Verification items for the finished model (mm, model axes). Face numbers are marked on the shaded views. A direction names the side the tool comes from. Give positions to 0.01 mm unless a question says otherwise; leave off trailing zeros. Order: outer loops, then holes, each group sorted by start corner. A loop starts at its lowest first (then second) coordinate and runs counter-clockwise, first axis right, second up. Notation, with made-up numbers: (66, 86.25) -> (82, 86.25) arc R27 cw to (82, 120.25) -> close; hole circle Ø8 at (67.25, 5.5). An arc over 180 degrees is marked (long way). Return JSON: item names as keys, results as strings. Group by question number.
(1) Cross-section at D-D on y = -50. Enter the section's corners in (x, z).
(2) Release check for a two-part mould opening along X. For the marked faces 1, 2 and 3 record: pulls with the +X half, pulls with the -X half, needs draft (parallel to the pull), parting line crosses it, or undercut.
(3) Cross-section at B-B on x = 0. Enter the section's corners in (y, z), then the cut area to 3 significant figures.
(4) Cross-section at C-C on z = -43. Enter the section's corners in (x, y), then the cut area to 3 significant figures.
(5) Thickness scan on line 1 along Y through (x, z) = (0, 1.5); line 2 along Z through (x, y) = (-19, 23.5); line 3 along Z through (x, y) = (17, 21). Record the ranges inside material, lowest first.
(6) Depth check by flat-ended pin: pin 1 Ø1.2 at (x, z) = (0, -43) entering from +Y; pin 2 Ø12 at (x, z) = (-18.5, -20.5) entering from -Y; pin 3 Ø8 at (x, z) = (15, -29.5) entering from +Y; pin 4 Ø11 at (x, y) = (7.5, 2.5) entering from +Z. Enter the tip coordinate at first touch or a pass-through.
(7) Cross-section at A-A on z = -1.5. Enter the section's corners in (x, y), then the cut area to 3 significant figures.
(8) Tool access check on the marked faces 4, 5, 6, 7 and 8. Record the directions out of +Z, -Z, +X, -X, +Y, -Y that give a thin tool (end or side, any length) a straight path to the whole face; none if there is none.
from build123d import *

# Parameters (mm, degrees)
F0_R      = 3.25
F1_DEPTH  = 50
F2_W      = 120.846782
F2_H      = 139.899194
F2_R      = 27.5
F3_DEPTH  = 45
F5_DEPTH  = 20
F7_DEPTH  = 10
F8_R      = 3.25
F8_R_2    = 27.5
F9_DEPTH  = 45
F10_W     = 122.298393
F10_H     = 98.165326
F10_R     = 5
F11_DEPTH = 20
F12_W     = 4
F12_H     = 52
F13_DEPTH = 20


with BuildPart() as f1:
    # F0 (on Top) → F1 (new body, symmetric)
    with BuildSketch(Plane.XY):
        with BuildLine():
            ThreePointArc((26.318053, -14.400002), (29.064941, -7.431635), (30, 0))
            ThreePointArc((30, 0), (29.064941, 7.431635), (26.318053, 14.400002))
            ThreePointArc((26.318053, 14.400002), (0, 30), (-26.318053, 14.400002))
            ThreePointArc((-26.318053, 14.400002), (-30, 0), (-26.318053, -14.400002))
            ThreePointArc((-26.318053, -14.400002), (0, -30), (26.318053, -14.400002))
        make_face()
        with BuildLine():
            ThreePointArc((-26.318053, 14.400002), (0, 30), (26.318053, 14.400002))
            Line((26.318053, 14.400002), (5.263611, 52.88))
            ThreePointArc((5.263611, 52.88), (5.812988, 51.486327), (6, 50))
            ThreePointArc((6, 50), (-1.486327, 44.187012), (-5.263611, 52.88))
            Line((-5.263611, 52.88), (-26.318053, 14.400002))
        make_face()
        with BuildLine():
            Line((5.263611, -52.88), (26.318053, -14.400002))
            ThreePointArc((26.318053, -14.400002), (0, -30), (-26.318053, -14.400002))
            Line((-26.318053, -14.400002), (-5.263611, -52.88))
            ThreePointArc((-5.263611, -52.88), (-1.486327, -44.187012), (6, -50))
            ThreePointArc((6, -50), (5.812988, -51.486327), (5.263611, -52.88))
        make_face()
        with BuildLine():
            ThreePointArc((6, 50), (5.812988, 51.486327), (5.263611, 52.88))
            ThreePointArc((5.263611, 52.88), (0, 56), (-5.263611, 52.88))
            ThreePointArc((-5.263611, 52.88), (-1.486327, 44.187012), (6, 50))
        make_face()
        with Locations((0, 50)):
            Circle(F0_R, mode=Mode.SUBTRACT)
        with BuildLine():
            ThreePointArc((-5.263611, -52.88), (0, -56), (5.263611, -52.88))
            ThreePointArc((5.263611, -52.88), (5.812988, -51.486327), (6, -50))
            ThreePointArc((6, -50), (-1.486327, -44.187012), (-5.263611, -52.88))
        make_face()
        with Locations((0, -50)):
            Circle(F0_R, mode=Mode.SUBTRACT)
    extrude(amount=F1_DEPTH, both=True)

    # F2 (on face) → F3 (cut)
    with BuildSketch(Plane.XY.offset(50)):
        with Locations((4.808469, 0)):
            Rectangle(F2_W, F2_H)
        Circle(F2_R, mode=Mode.SUBTRACT)
    extrude(amount=-F3_DEPTH, mode=Mode.SUBTRACT)

    # F4 (on face) → F5 (cut)
    with BuildSketch(Plane.XY.offset(50)):
        with BuildLine():
            Line((-2.5, 16.312995), (-2.5, 38.387493))
            ThreePointArc((-2.5, 38.387493), (-38.468814, 0), (-2.5, -38.387493))
            Line((-2.5, -38.387493), (-2.5, -16.312995))
            ThreePointArc((-2.5, -16.312995), (-16.503448, 0), (-2.5, 16.312995))
        make_face()
        with BuildLine():
            ThreePointArc((2.5, -38.387493), (38.468814, 0), (2.5, 38.387493))
            Line((2.5, 38.387493), (2.5, 16.312995))
            ThreePointArc((2.5, 16.312995), (16.503448, 0), (2.5, -16.312995))
            Line((2.5, -16.312995), (2.5, -38.387493))
        make_face()
    extrude(amount=-F5_DEPTH, mode=Mode.SUBTRACT)

    # F6 (on face) → F7 (cut)
    with BuildSketch(Plane.XY.offset(50)):
        with BuildLine():
            ThreePointArc((2.5, 5.454356), (5.049752, 3.24037), (6, 0))
            ThreePointArc((6, 0), (5.049752, -3.24037), (2.5, -5.454356))
            Line((2.5, -5.454356), (2.5, -22.150979))
            ThreePointArc((2.5, -22.150979), (22.29161, 0), (2.5, 22.150979))
            Line((2.5, 22.150979), (2.5, 5.454356))
        make_face()
        with BuildLine():
            ThreePointArc((-2.5, -5.454356), (-6, 0), (-2.5, 5.454356))
            Line((-2.5, 5.454356), (-2.5, 22.150979))
            ThreePointArc((-2.5, 22.150979), (-22.29161, 0), (-2.5, -22.150979))
            Line((-2.5, -22.150979), (-2.5, -5.454356))
        make_face()
        with BuildLine():
            ThreePointArc((-2.5, -16.312995), (-16.503448, 0), (-2.5, 16.312995))
            Line((-2.5, 16.312995), (-2.5, 22.150979))
            ThreePointArc((-2.5, 22.150979), (-22.29161, 0), (-2.5, -22.150979))
            Line((-2.5, -22.150979), (-2.5, -16.312995))
        make_face()
        with BuildLine():
            Line((2.5, 22.150979), (2.5, 16.312995))
            ThreePointArc((2.5, 16.312995), (16.503448, 0), (2.5, -16.312995))
            Line((2.5, -16.312995), (2.5, -22.150979))
            ThreePointArc((2.5, -22.150979), (22.29161, 0), (2.5, 22.150979))
        make_face()
    extrude(amount=-F7_DEPTH, mode=Mode.SUBTRACT)

    # F8 (on face) → F9 (cut)
    with BuildSketch(Plane(origin=(0, 0, -50), x_dir=(1, 0, 0), z_dir=(0, 0, -1))):
        with BuildLine():
            Line((5.263611, -52.88), (26.318053, -14.400002))
            ThreePointArc((26.318053, -14.400002), (30, 0), (26.318053, 14.400002))
            Line((26.318053, 14.400002), (5.263611, 52.88))
            ThreePointArc((5.263611, 52.88), (0, 56), (-5.263611, 52.88))
            Line((-5.263611, 52.88), (-26.318053, 14.400002))
            ThreePointArc((-26.318053, 14.400002), (-30, 0), (-26.318053, -14.400002))
            Line((-26.318053, -14.400002), (-5.263611, -52.88))
            ThreePointArc((-5.263611, -52.88), (0, -56), (5.263611, -52.88))
        make_face()
        with Locations((0, -50)):
            Circle(F8_R, mode=Mode.SUBTRACT)
        Circle(F8_R_2, mode=Mode.SUBTRACT)
        with Locations((0, 50)):
            Circle(F8_R, mode=Mode.SUBTRACT)
    extrude(amount=-F9_DEPTH, mode=Mode.SUBTRACT)

    # F10 (on face) → F11 (cut)
    with BuildSketch(Plane(origin=(0, 0, -50), x_dir=(1, 0, 0), z_dir=(0, 0, -1))):
        with Locations((4.808468, -5.987905)):
            Rectangle(F10_W, F10_H)
        with Locations((-15, 0)):
            Circle(F10_R, mode=Mode.SUBTRACT)
        with Locations((15, 0)):
            Circle(F10_R, mode=Mode.SUBTRACT)
    extrude(amount=-F11_DEPTH, mode=Mode.SUBTRACT)

    # F12 (on face) → F13 (join)
    with BuildSketch(Plane(origin=(0, 0, -30), x_dir=(1, 0, 0), z_dir=(0, 0, -1))):
        Rectangle(F12_W, F12_H)
    extrude(amount=F13_DEPTH)


solid = f1.part
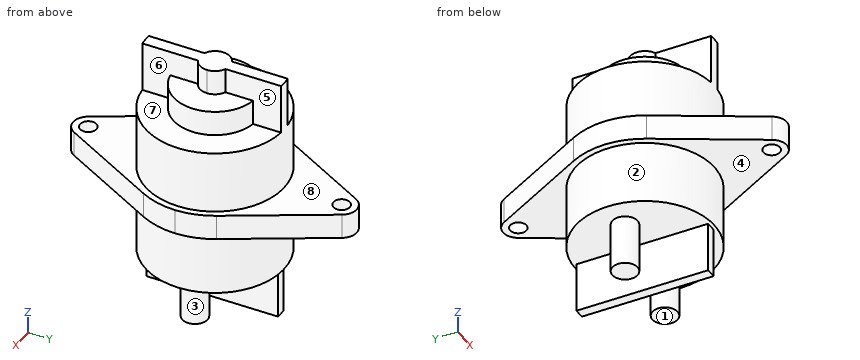
Verdict:
{
 "1": {"outline": "(-6.84, -5) -> (-3.25, -5) -> (-3.25, 5) -> (-6.84, 5) -> close; (3.25, -5) -> (6.84, -5) -> (6.84, 5) -> (3.25, 5) -> close"},
 "2": {"face 1": "needs draft", "face 2": "parting line crosses it", "face 3": "undercut"},
 "3": {"outline": "(-56, -5) -> (-53.25, -5) -> (-53.25, 5) -> (-56, 5) -> close; (-46.75, -5) -> (-27.5, -5) -> (-27.5, -30) -> (-26, -30) -> (-26, -50) -> (26, -50) -> (26, -30) -> (27.5, -30) -> (27.5, -5) -> (46.75, -5) -> (46.75, 5) -> (27.5, 5) -> (27.5, 50) -> (-27.5, 50) -> (-27.5, 5) -> (-46.75, 5) -> close; (53.25, -5) -> (56, -5) -> (56, 5) -> (53.25, 5) -> close", "area": "5,880 mm²"},
 "4": {"outline": "circle Ø10 at (-15, 0); (-2, -26) -> (2, -26) -> (2, 26) -> (-2, 26) -> close; circle Ø10 at (15, 0)", "area": "365 mm²"},
 "5": {"line 1": "-56 to -53.25, -46.75 to 46.75, 53.25 to 56", "line 2": "-5 to 5", "line 3": "-30 to 30"},
 "6": {"pin 1": "y = 26", "pin 2": "y = -24.49", "pin 3": "y = 25.2", "pin 4": "z = 50"},
 "7": {"outline": "(-26.32, -14.4) -> (-5.26, -52.88) arc R6 ccw to (5.26, -52.88) -> (26.32, -14.4) arc R30 ccw to (26.32, 14.4) -> (5.26, 52.88) arc R6 ccw to (-5.26, 52.88) -> (-26.32, 14.4) arc R30 ccw to start; hole circle Ø6.5 at (0, -50); hole circle Ø6.5 at (0, 50)", "area": "4,070 mm²"},
 "8": {"face 4": "-Z", "face 5": "+Z, +X, +Y", "face 6": "+Z, +X, -Y", "face 7": "+Z, +X", "face 8": "+Z"}
}
